```python
from build123d import *

# Parameters (mm, degrees)
SKETCH4_R               = 7.5
SKETCH1_R               = 8.5
SKETCH5_W               = 13.984772719
SKETCH5_H               = 8.5
CUT_EXTRUDE1_DEPTH      = 10
CUT_EXTRUDE1_DEPTH_BACK = 10
CUT_EXTRUDE2_DEPTH      = 10
CUT_EXTRUDE2_DEPTH_BACK = 10
SKETCH8_R               = 1.25
CUT_EXTRUDE3_DEPTH      = 10
CUT_EXTRUDE3_DEPTH_BACK = 10
CUT_EXTRUDE4_DEPTH      = 12
FILLET1_R               = 1


with BuildPart() as part:
    # Sketch4 → Loft1 section 0
    with BuildSketch(Plane(origin=(-22, 0, 0), x_dir=(0, 0, -1), z_dir=(1, 0, 0))):
        Circle(SKETCH4_R)
    # Sketch1 → Loft1 section 1
    with BuildSketch(Plane(origin=(0, 0, 0), x_dir=(0, 0, -1), z_dir=(1, 0, 0))):
        Circle(SKETCH1_R)
    loft()

    # Sketch5 → Cut-Extrude1 (cut, two sides)
    with BuildSketch(Plane.XY) as cut_extrude1_sk:
        with Locations((-17.99238636, 0)):
            Rectangle(SKETCH5_W, SKETCH5_H)
    extrude(amount=CUT_EXTRUDE1_DEPTH, mode=Mode.SUBTRACT)
    extrude(cut_extrude1_sk.sketch, amount=-CUT_EXTRUDE1_DEPTH_BACK, mode=Mode.SUBTRACT)

    # Sketch7 → Cut-Extrude2 (cut, two sides)
    with BuildSketch(Plane(origin=(0, 0, 0), x_dir=(1, 0, 0), z_dir=(0, 1, 0))) as cut_extrude2_sk:
        with BuildLine():
            ThreePointArc((-16.527422763, 6.684642149), (-21.211826581, 3.739953342), (-23.023054805, -1.488266586))
            Line((-23.023054805, -1.488266586), (-23.002284576, -6.042868806))
            Line((-23.002284576, -6.042868806), (-11, -6.777720856))
            Line((-11, -6.777720856), (-11, -8.501479668))
            Line((-11, -8.501479668), (-27.91814199, -8.501479668))
            Line((-27.91814199, -8.501479668), (-27.91814199, 10.370496294))
            Line((-27.91814199, 10.370496294), (-11, 10.370496294))
            Line((-11, 10.370496294), (-11, 6.777720856))
            Line((-11, 6.777720856), (-16.527422763, 6.684642149))
        make_face()
    extrude(amount=CUT_EXTRUDE2_DEPTH, mode=Mode.SUBTRACT)
    extrude(cut_extrude2_sk.sketch, amount=-CUT_EXTRUDE2_DEPTH_BACK, mode=Mode.SUBTRACT)

    # Sketch8 → Cut-Extrude3 (cut, two sides)
    with BuildSketch(Plane(origin=(0, 0, 0), x_dir=(1, 0, 0), z_dir=(0, 1, 0))) as cut_extrude3_sk:
        with Locations((-15.3, 0.5)):
            Circle(SKETCH8_R)
    extrude(amount=CUT_EXTRUDE3_DEPTH, mode=Mode.SUBTRACT)
    extrude(cut_extrude3_sk.sketch, amount=-CUT_EXTRUDE3_DEPTH_BACK, mode=Mode.SUBTRACT)

    # Sketch10 → Cut-Extrude4 (cut)
    with BuildSketch(Plane(origin=(0, 0, 0), x_dir=(0, 0, -1), z_dir=(1, 0, 0))):
        with BuildLine():
            Line((-4.5, 4.25), (4.5, 4.25))
            ThreePointArc((4.5, 4.25), (5.331033358, -0.026207333), (4.26513416, -4.25))
            Line((4.26513416, -4.25), (-4.73486584, -4.25))
            ThreePointArc((-4.73486584, -4.25), (-5.565899198, 0.026207333), (-4.5, 4.25))
        make_face()
    extrude(amount=-CUT_EXTRUDE4_DEPTH, mode=Mode.SUBTRACT)

    # Fillet1
    fillet1_edges = [part.edges().sort_by_distance(p)[0] for p in [
        (-22, -4.303779405, 6.104234696),
        (-22, 4.303779405, 6.104234696),
    ]]
    fillet(fillet1_edges, radius=FILLET1_R)


solid = part.part
```
CAD build for the part. Positions are in the model's coordinates, mm. A direction names the side the tool comes from. Round coordinates to 2 decimals unless told otherwise and drop trailing zeros. Order: outer loops, then holes, each group sorted by start corner. A loop starts at its lowest first (then second) coordinate and runs counter-clockwise, first axis right, second up. Notation, with made-up numbers: (80.25, 14.5) - (139.25, 14.5) arc R23 cw to (139.25, 33.5) - close; hole circle Ø8 at (27, 40.25). An arc over 180 degrees is marked (long way). Answer as CSV lines item,"result". Start each with the question number.
1. Saw through at C-C, the plane x = -15.3. Write the cut outline in (y, z), and give its area (3 significant figures).
2. Drill centre lines: L1, parallel to X at y = 5.7, z = -0.5; L2, parallel to Z at x = -9.75, y = 0.75; L3, parallel to Y at x = -13, z = -4.75. Where is each one in solid material? Low to high. Write a range as [from, to].
3. Pull direction Z, two halves, no side cores. Call faces 5 (the face through (-21.9, 4.6, 5.6)), 6 (the face through (-22, -6, 1)), 7 (the face through (-14.723, -6.029, 0.609)), 8 (the face through (-20.54, 5.32, -4.49)): +Z half, -Z half, draft (parallel to the pull), parting line (faces both ways), or undercut.
4. Saw through at B-B, the plane z = 0. Write the cut outline in (x, y), and give its area (3 significant figures).
5. Pin check, flat tips, straight feed: pin 1 (6 mm diameter, centred on y = -3, z = 1, fed in from -X); pin 2 (2 mm diameter, centred on x = -8.5, y = 2, fed in from -Z); pin 3 (5 mm diameter, centred on x = -4.5, y = 0.5, fed in from -Z); pin 4 (1 mm diameter, centred on y = -2, z = 6.5, fed in from -X). Stop position of each tip, or through.
6. Tool access for faces 1 (the face through (-14.723, 6.029, 0.609)), 2 (the face through (-5.423, 0.035, -5.333)), 3 (the face through (-11, 0, 7)), 4 (the face through (-11, 4.25, 0)): list every direction of +Z, -Z, +X, -X, +Y, -Y with a clear straight run to the whole face (end or side of a thin tool).
Model answer:
1,outline,"(-7.77, 0.75) - (-4.25, 0.75) - (-4.25, 6.51) - (-4.3, 6.51) arc R7.8 ccw to start; (-7.61, -1.75) arc R7.8 ccw to (-4.25, -6.55) - (-4.25, -1.75) - close; (4.25, -6.55) arc R7.8 ccw to (7.61, -1.75) - (4.25, -1.75) - close; (4.25, 0.75) - (7.77, 0.75) arc R7.8 ccw to (4.3, 6.51) - (4.25, 6.51) - close"
1,area,"48.0 mm²"
2,L1,"x = [-22, -16.55], [-14.05, 0]"
2,L2,"z = [-8.02, -5.32], [5.52, 8.02]"
2,L3,"y = [-6.32, -4.25], [4.25, 6.32]"
3,face 5,"+Z half"
3,face 6,"draft"
3,face 7,"undercut"
3,face 8,"-Z half"
4,outline,"(-22, -7.5) - (-16.45, -7.75) - (-16.45, -4.25) - (-22, -4.25) - close; (-22, 4.25) - (-16.45, 4.25) - (-16.45, 7.75) - (-22, 7.5) - close; (-14.15, -7.86) - (0, -8.5) - (0, -4.25) - (-14.15, -4.25) - close; (-14.15, 4.25) - (0, 4.25) - (0, 8.5) - (-14.15, 7.86) - close"
4,area,"149 mm²"
5,pin 1,"stops at x = -22"
5,pin 2,"stops at z = -8.06"
5,pin 3,"stops at z = -8.41"
5,pin 4,"stops at x = -11"
6,face 1,"+Y, -Y"
6,face 2,"+X, -X"
6,face 3,"+Z, -Z, -X"
6,face 4,"-X"
